Can you work these out from the model? Positions are in its coordinate system, mm. A direction names the side the tool comes from. Coordinates: 2 decimals unless noted, no trailing zeros. Loops run counter-clockwise (first coordinate to the right, second up) from the corner with the lowest first, then second, coordinate; pieces in that order, holes last.
```python
from build123d import *

# Parameters (mm, degrees)
SKETCH1_W           = 7
SKETCH1_H           = 7
BOSS_EXTRUDE1_DEPTH = 3
CUT_EXTRUDE1_DEPTH  = 7
CUT_EXTRUDE2_DEPTH  = 11
SKETCH4_R           = 1.8
CUT_EXTRUDE3_DEPTH  = 0.8
CUT_EXTRUDE4_DEPTH  = 0.4


with BuildPart() as part:
    # Sketch1 → Boss-Extrude1 (new body)
    with BuildSketch(Plane(origin=(0, 0, 0), x_dir=(1, 0, 0), z_dir=(0, 1, 0))):
        with Locations((3.5, 3.5)):
            Rectangle(SKETCH1_W, SKETCH1_H)
    extrude(amount=BOSS_EXTRUDE1_DEPTH)

    # Sketch2 → Cut-Extrude1 (cut)
    with BuildSketch(Plane.XY):
        Polygon((0, 0), (0.7, 3), (0, 3), align=None)
        Polygon((7, 0), (6.3, 3), (7, 3), align=None)
    extrude(amount=-CUT_EXTRUDE1_DEPTH, mode=Mode.SUBTRACT)

    # Sketch3 → Cut-Extrude2 (cut)
    with BuildSketch(Plane(origin=(0, 0, 0), x_dir=(0, 0, -1), z_dir=(1, 0, 0))):
        Polygon((0, 0), (0.7, 3), (0, 3), align=None)
        Polygon((7, 3), (6.3, 3), (7, 0), align=None)
    extrude(amount=CUT_EXTRUDE2_DEPTH, mode=Mode.SUBTRACT)

    # Sketch4 → Cut-Extrude3 (cut)
    with BuildSketch(Plane.XZ):
        with Locations(Location((3.5, -3.5, 0), (0, 0, 270))):
            Circle(SKETCH4_R)
    extrude(amount=-CUT_EXTRUDE3_DEPTH, mode=Mode.SUBTRACT)

    # Sketch5 → Cut-Extrude4 (cut)
    with BuildSketch(Plane(origin=(0, 3, 0), x_dir=(1, 0, 0), z_dir=(0, 1, 0))):
        with BuildLine():
            Line((3.074992012, 4.468285429), (4.036530474, 4.468285429))
            Line((4.036530474, 4.468285429), (4.036530474, 3.769166839))
            add(Edge.make_bspline(
                [(4.036530474, 3.769166839), (4.036086851, 3.702022613), (4.035249234, 3.575245505), (4.020566764, 3.39640898), (4.000165605, 3.239359877), (3.967710391, 3.102079519), (3.924256019, 2.978103986), (3.862818552, 2.864662172), (3.787262222, 2.756102323), (3.694844376, 2.655709349), (3.588530384, 2.562855929), (3.467088334, 2.482109847), (3.333400229, 2.410169074), (3.237355705, 2.372295276), (3.188173102, 2.352900814)],
                knots=[0, 0, 0, 0, 1.347156832, 2.543608823, 3.599300285, 4.522475688, 5.370350604, 6.227678973, 7.103274953, 8.018757603, 8.959280198, 9.929437417, 10.939703653, 12, 12, 12, 12], degree=3))
            Line((3.188173102, 2.352900814), (3.010889448, 2.737516198))
            add(Edge.make_bspline(
                [(3.010889448, 2.737516198), (3.053777828, 2.755154018), (3.135615846, 2.78880985), (3.245316967, 2.853643094), (3.334062536, 2.929935998), (3.405416723, 3.016399576), (3.45643151, 3.118107137), (3.494770079, 3.233341119), (3.516994248, 3.365049182), (3.521395894, 3.457921451), (3.523709961, 3.506746968)],
                knots=[0, 0, 0, 0, 1.113959817, 2.125616841, 3.047494432, 3.914868512, 4.801521967, 5.765947312, 6.825496818, 8, 8, 8, 8], degree=3))
            Line((3.523709961, 3.506746968), (3.074992012, 3.506746968))
            Line((3.074992012, 3.506746968), (3.074992012, 4.468285429))
        make_face()
    extrude(amount=-CUT_EXTRUDE4_DEPTH, mode=Mode.SUBTRACT)


solid = part.part
```
Item 1: Suppose I cut it at B-B, the plane x = 1. Please give me the cut outline in (y, z).
Results are:
outline: (0, -7) - (3, -6.3) - (3, -0.7) - (0, 0) - close
Item 2: Suppose I cut it at C-C, the plane y = 1.7. Please give me the cut outline in (x, z), plus the area to 3 significant figures.
Results are:
outline: (0.4, -6.6) - (6.6, -6.6) - (6.6, -0.4) - (0.4, -0.4) - close
area: 38.5 mm2
Item 3: Suppose I cut it at D-D, the plane x = 4.25. Please give me the cut outline in (y, z).
Results are:
outline: (0, -7) - (3, -6.3) - (3, -0.7) - (0, 0) - (0, -1.86) - (0.8, -1.86) - (0.8, -5.14) - (0, -5.14) - close
Item 4: We'd pull the mould along X, two halves only. Please class faces 1 (the face through (3.451, 1.521, -6.645)), 2 (the face through (6.655, 1.479, -3.451)), 3 (the face through (0.345, 1.479, -3.451)), 4 (the face through (4.041, 0.394, -5.217)): +X half, -X half, draft (parallel to the pull), parting line (faces both ways), or undercut.
Results are:
face 1: draft
face 2: +X half
face 3: -X half
face 4: undercut
Item 5: Suppose I cut it at A-A, the plane z = -2. Please give me the cut outline in (x, y), plus the area to 3 significant figures.
Results are:
outline: (0, 0) - (2.51, 0) - (2.51, 0.8) - (4.49, 0.8) - (4.49, 0) - (7, 0) - (6.3, 3) - (0.7, 3) - close
area: 17.3 mm2
Item 6: On a 3-axis mill with a long thin cutter (end or side, diameter ignored), from which of +Z, -Z, +X, -X, +Y, -Y can I reach the whole of each face in a straight line? I mean faces 5 (the face through (3.451, 1.479, -0.345)), 6 (the face through (4, 0.8, -3)). Say none if no direction works.
Results are:
face 5: +Z, +X, -X, +Y
face 6: -Y
Item 7: I need wall thicknesses on line 1 along X through (y, z) = (0.65, -3.5); line 2 along X through (y, z) = (0.6, -3.5); line 3 along Z through (x, y) = (3.25, 0.35). Which ranges of each line are inside material? Lowest first, please.
Results are:
line 1: x = 0.15 to 1.7, 5.3 to 6.85
line 2: x = 0.14 to 1.7, 5.3 to 6.86
line 3: z = -6.92 to -5.28, -1.72 to -0.08
Item 8: I'm going to push flat-ended pins straight in: P1, Ø1.8, axis at x = 3.5, z = -4, coming from the -Y side; P2, Ø1, axis at y = 1.5, z = -3, coming from the -X side; P3, Ø1.5, axis at x = 6, y = 2, coming from the +Z side. Where does each tip first touch, or does it pass through?
Results are:
P1: stops at y = 0.8
P2: stops at x = 0.23
P3: stops at z = -0.29
